CAD build for the part. Positions are in the model's coordinates, mm. A direction names the side the tool comes from. Coordinates: 2 decimals unless noted, no trailing zeros. Loops run counter-clockwise (first coordinate to the right, second up) from the corner with the lowest first, then second, coordinate; pieces in that order, holes last. Notation, with made-up numbers: (22.5, 61.5) - (43.5, 61.5) arc R21 cw to (43.5, 83.5) - close; hole circle Ø7 at (80, -8.5). An arc over 180 degrees is marked (long way). Put each result on its own line as item: value.
```python
from build123d import *

# Parameters (mm, degrees)
EXTRUDE004_DEPTH      = 20
EXTRUDE001_DEPTH      = 5
SKETCH002_R           = 57.15
SKETCH002_R_2         = 47.15
EXTRUDE002_DEPTH      = 270
EXTRUDE003_DEPTH      = 5
CLONE_PLACEMENT_ANGLE = 180
SKETCH_W              = 300
SKETCH_H              = 160
SKETCH_R              = 9
EXTRUDE_DEPTH         = 30


with BuildPart() as lastplatte:
    # Sketch004 (on Face26 of Fusion) → Extrude004 (new body)
    with BuildSketch(Plane.XY.offset(300)):
        Polygon((65, 37.527767), (0, 75.055535), (-65, 37.527767), (-65, -37.527767), (0, -75.055535), (65, -37.527767), align=None)
    extrude(amount=-EXTRUDE004_DEPTH)


with BuildPart() as obj1:
    # Sketch001 → Extrude001 (new body, symmetric)
    with BuildSketch(Plane.XZ):
        Polygon((150, 30), (-150, 30), (-150, 80), (-100, 130), (100, 130), (150, 80), align=None)
    extrude(amount=EXTRUDE001_DEPTH, both=True)


with BuildPart() as obj2:
    # Sketch002 (on Face10 of Extrude) → Extrude002 (new body)
    with BuildSketch(Plane.XY.offset(30)):
        Circle(SKETCH002_R)
        Circle(SKETCH002_R_2, mode=Mode.SUBTRACT)
    extrude(amount=EXTRUDE002_DEPTH)


with BuildPart() as obj3:
    # Sketch003 → Extrude003 (new body, symmetric)
    with BuildSketch(Plane.YZ):
        Polygon((-80, 30), (-80, 80), (-65, 130), (-5, 130), (-5, 30), align=None)
    extrude(amount=EXTRUDE003_DEPTH, both=True)


with BuildPart() as obj4:
    # Clone base: copy of obj3
    add(obj3.part)


with BuildPart() as obj4_1:
    # Clone placement: moved
    add(obj4.part.rotate(Axis((0, 0, 0), (0, 0, 1)), CLONE_PLACEMENT_ANGLE))


with BuildPart() as fusion001:
    # Sketch → Extrude (new body)
    with BuildSketch(Plane.XY):
        Rectangle(SKETCH_W, SKETCH_H)
        with Locations((-120, 50)):
            Circle(SKETCH_R, mode=Mode.SUBTRACT)
        with Locations((120, 50)):
            Circle(SKETCH_R, mode=Mode.SUBTRACT)
        with Locations((120, -50)):
            Circle(SKETCH_R, mode=Mode.SUBTRACT)
        with Locations((-120, -50)):
            Circle(SKETCH_R, mode=Mode.SUBTRACT)
    extrude(amount=EXTRUDE_DEPTH)

    # Fusion: union obj1, obj2, obj3, obj4
    add(obj1.part)
    add(obj2.part)
    add(obj3.part)
    add(obj4_1.part)

    # Fusion001: union lastplatte
    add(lastplatte.part)


solid = fusion001.part
```
Q1. Wall check: L1, parallel to Y at x = -120, z = 22; L2, parallel to X at y = 24, z = 114; L3, parallel to Y at x = -2, z = 234.5 (3 decimals). Give the ranges that are in metal, low to high. Write a range as from..to.
Determined:
L1: -80..-59, -41..41, 59..80
L2: -51.87..-40.58, -5..5, 40.58..51.87
L3: -57.115..-47.108, 47.108..57.115
Q2. Mould opens along Y. For faces 5 (the flat face through (-150, -1, 22)), 6 (the flat face through (-0.07, 72.605, 104.65)), 7 (the flat face through (-26, 5, 81)) say: +Y half, -Y half, draft (parallel to the pull), parting line (faces both ways), or undercut.
Determined:
face 5: draft
face 6: +Y half
face 7: undercut
Q3. Tool access for faces 1 (the flat face through (-32.95, -56.03, 290.14)), 2 (the flat face through (-95, 43, 30)), 3 (the flat face through (-95, -42, 30)), 4 (the flat face through (-1, 1, 280)): list every direction of +Z, -Z, +X, -X, +Y, -Y with a clear straight run to the whole face (end or side of a thin tool).
Determined:
face 1: +Z, -X, -Y
face 2: -X, +Y
face 3: -X, -Y
face 4: none
Q4. Slice it at A-A, the plane x = 120. Give the cut face in (y, z).
Determined:
outline: (-80, 0) - (-59, 0) - (-59, 30) - (-80, 30) - close; (-41, 0) - (41, 0) - (41, 30) - (5, 30) - (5, 110) - (-5, 110) - (-5, 30) - (-41, 30) - close; (59, 0) - (80, 0) - (80, 30) - (59, 30) - close
Q5. Slice it at B-B, the plane z = 96.5. Give the cut face in (x, y).
Determined:
outline: (-133.5, -5) - (-56.93, -5) arc R57.15 ccw to (-5, -56.93) - (-5, -75.05) - (5, -75.05) - (5, -56.93) arc R57.15 ccw to (56.93, -5) - (133.5, -5) - (133.5, 5) - (56.93, 5) arc R57.15 ccw to (5, 56.93) - (5, 75.05) - (-5, 75.05) - (-5, 56.93) arc R57.15 ccw to (-56.93, 5) - (-133.5, 5) - close; hole (-46.88, -5) arc R47.15 ccw to (-5, -46.88) - (-5, -5) - close; hole (-46.88, 5) - (-5, 5) - (-5, 46.88) arc R47.15 ccw to start; hole (5, -46.88) arc R47.15 ccw to (46.88, -5) - (5, -5) - close; hole (5, 5) - (46.88, 5) arc R47.15 ccw to (5, 46.88) - close
Q6. Slice it at D-D, the plane z = 239. Give the cut face in (x, y), then the cut area to 3 significant figures.
Determined:
outline: circle Ø114.3 at (0, 0); hole circle Ø94.3 at (0, 0)
area: 3,280 mm2
Q7. Pin check, flat tips, straight feed: pin 1 Ø10 at (x, y) = (-49.5, -47) entering from -Z; pin 2 Ø5 at (y, z) = (-14, 138) entering from -X; pin 3 Ø21 at (x, z) = (16.5, 70.5) entering from -Y; pin 4 Ø8 at (y, z) = (-23.5, 228.5) entering from +X. Stop position of each tip, or through.
Determined:
pin 1: z = 0
pin 2: x = -55.98
pin 3: y = -56.83
pin 4: x = 53.72
Q8. Slice it at C-C, the plane y = 0. Give the cut face in (x, z), then the cut area to 3 significant figures.
Determined:
outline: (-150, 0) - (150, 0) - (150, 80) - (100, 130) - (57.15, 130) - (57.15, 280) - (65, 280) - (65, 300) - (-65, 300) - (-65, 280) - (-57.15, 280) - (-57.15, 130) - (-100, 130) - (-150, 80) - close; hole (-47.15, 130) - (47.15, 130) - (47.15, 280) - (-47.15, 280) - close
area: 42,100 mm2
